Check sheet for the modelled part. Datum: model origin and axes. Units: mm. Face numbers are marked on the shaded views. A direction names the side the tool comes from. Round coordinates to 2 decimals unless told otherwise and drop trailing zeros. Write each loop counter-clockwise with the first axis right and the second up, starting at its lowest first coordinate (ties: lowest second). Pieces come first, ordered by that corner, then holes. Notation, with made-up numbers: M -22,18.25 L 24,18.25 A19 ccw 24,55.25 Z; hole C -37.75,54 d9. An arc over 180 degrees is marked long. Answer in a Markdown table with one row per item.
```python
from build123d import *

# Parameters (mm, degrees)
SKETCH_1_W          = 75
SKETCH_1_H          = 40
EXTRUDE_1_DEPTH     = 18
CHAMFER_1_SIZE      = 5
SKETCH_2_W          = 45
SKETCH_2_H          = 10
EXTRUDE_2_DEPTH     = 44.5
CHAMFER_2_SIZE      = 5
SKETCH_3_R          = 17.5
CUT_EXTRUDE_1_DEPTH = 101.778221854
SKETCH_4_R          = 1.5
CUT_EXTRUDE_2_DEPTH = 101.778221854
SKETCH_5_R          = 5
CUT_EXTRUDE_3_DEPTH = 6
SKETCH_6_R          = 2.75
CUT_EXTRUDE_4_DEPTH = 99.869863963


with BuildPart() as part:
    # 스케치1 → 보스-돌출1 (new body)
    with BuildSketch(Plane(origin=(0, 0, 0), x_dir=(1, 0, 0), z_dir=(0, 1, 0))):
        with Locations((37.5, 20)):
            Rectangle(SKETCH_1_W, SKETCH_1_H)
    extrude(amount=EXTRUDE_1_DEPTH)

    # 모따기1
    chamfer_1_edges = [part.edges().sort_by_distance(p)[0] for p in [
        (0, 9, -40),
        (75, 9, -40),
        (75, 9, 0),
        (0, 9, 0),
    ]]
    chamfer(chamfer_1_edges, length=CHAMFER_1_SIZE)

    # 스케치2 → 보스-돌출2 (add)
    with BuildSketch(Plane(origin=(0, 18, 0), x_dir=(1, 0, 0), z_dir=(0, 1, 0))):
        with Locations((37.5, 20)):
            Rectangle(SKETCH_2_W, SKETCH_2_H)
    extrude(amount=EXTRUDE_2_DEPTH)

    # 모따기2
    chamfer_2_edges = [part.edges().sort_by_distance(p)[0] for p in [
        (15, 62.5, -20),
        (60, 62.5, -20),
    ]]
    chamfer(chamfer_2_edges, length=CHAMFER_2_SIZE)

    # 스케치3 → 컷-돌출1 (cut, through all)
    with BuildSketch(Plane.XY.offset(-15)):
        with Locations((37.5, 40)):
            Circle(SKETCH_3_R)
    extrude(amount=-CUT_EXTRUDE_1_DEPTH, mode=Mode.SUBTRACT)

    # 스케치4 → 컷-돌출2 (cut, through all)
    with BuildSketch(Plane.XY.offset(-15)):
        with Locations((22.65, 54.85)):
            Circle(SKETCH_4_R)
        with Locations((52.35, 54.85)):
            Circle(SKETCH_4_R)
        with Locations((52.35, 25.15)):
            Circle(SKETCH_4_R)
        with Locations((22.65, 25.15)):
            Circle(SKETCH_4_R)
    extrude(amount=-CUT_EXTRUDE_2_DEPTH, mode=Mode.SUBTRACT)

    # 스케치5 → 컷-돌출3 (cut)
    with BuildSketch(Plane(origin=(0, 18, 0), x_dir=(1, 0, 0), z_dir=(0, 1, 0))):
        with Locations(Location((10, 32.5, 0), (0, 0, 270))):
            Circle(SKETCH_5_R)
        with Locations(Location((10, 7.5, 0), (0, 0, 270))):
            Circle(SKETCH_5_R)
        with Locations(Location((65, 7.5, 0), (0, 0, 270))):
            Circle(SKETCH_5_R)
        with Locations(Location((65, 32.5, 0), (0, 0, 270))):
            Circle(SKETCH_5_R)
    extrude(amount=-CUT_EXTRUDE_3_DEPTH, mode=Mode.SUBTRACT)

    # 스케치6 → 컷-돌출4 (cut, through all)
    with BuildSketch(Plane(origin=(0, 12, 0), x_dir=(1, 0, 0), z_dir=(0, 1, 0))):
        with Locations(Location((10, 7.5, 0), (0, 0, 270))):
            Circle(SKETCH_6_R)
        with Locations(Location((10, 32.5, 0), (0, 0, 270))):
            Circle(SKETCH_6_R)
        with Locations(Location((65, 7.5, 0), (0, 0, 270))):
            Circle(SKETCH_6_R)
        with Locations(Location((65, 32.5, 0), (0, 0, 270))):
            Circle(SKETCH_6_R)
    extrude(amount=-CUT_EXTRUDE_4_DEPTH, mode=Mode.SUBTRACT)


solid = part.part
```
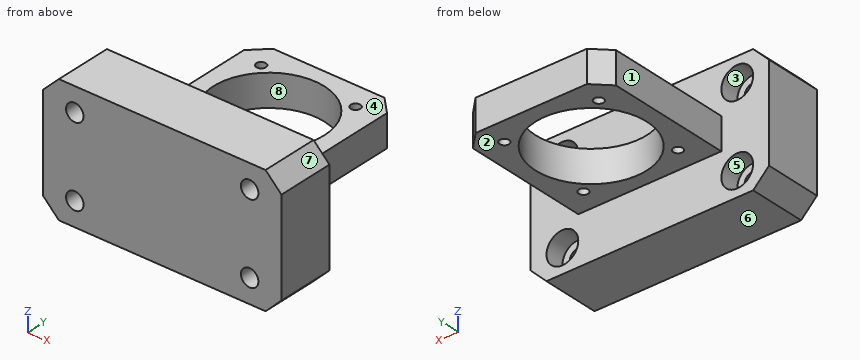
1. Access from +Z, -Z, +X, -X, +Y, -Y to the whole of each face (thin tool, end or side, straight path). Record for the marked faces 1, 2, 3 and 4.
Found:
| item | result |
|---|---|
| face 1 | +Z, -Z, -X, +Y |
| face 2 | -Z, +X, -X, +Y |
| face 3 | +Y |
| face 4 | +Z, +X, -X, +Y |
2. Section check C-C, the plane x = 10. Record the cut outline in (y, z).
Found:
| item | result |
|---|---|
| outline | M 0,-40 L 18,-40 L 18,-37.5 L 12,-37.5 L 12,-35.25 L 0,-35.25 Z; M 0,-29.75 L 12,-29.75 L 12,-27.5 L 18,-27.5 L 18,-12.5 L 12,-12.5 L 12,-10.25 L 0,-10.25 Z; M 0,-4.75 L 12,-4.75 L 12,-2.5 L 18,-2.5 L 18,0 L 0,0 Z |
3. Section check A-A, the plane y = 40. Record the cut outline in (x, z), and give its area (3 significant figures).
Found:
| item | result |
|---|---|
| outline | M 15,-25 L 20,-25 L 20,-15 L 15,-15 Z; M 55,-25 L 60,-25 L 60,-15 L 55,-15 Z |
| area | 100 mm2 |
4. Go/stop test with flat-tipped pins: pin 1 (5 mm diameter, centred on x = 22.65, y = 54.85, fed in from -Z); pin 2 (3 mm diameter, centred on y = 43, z = -20.5, fed in from -X); pin 3 (11 mm diameter, centred on x = 8.5, z = -32, fed in from +Y); pin 4 (1.8 mm diameter, centred on x = 22.65, y = 25.15, fed in from -Z). Record where each tip stops, or that it passes through.
Found:
| item | result |
|---|---|
| pin 1 | stops at z = -25 |
| pin 2 | stops at x = 15 |
| pin 3 | stops at y = 18 |
| pin 4 | passes through |
5. Section check D-D, the plane y = 14. Record the cut outline in (x, z).
Found:
| item | result |
|---|---|
| outline | M 0,-35 L 5,-40 L 70,-40 L 75,-35 L 75,-5 L 70,0 L 5,0 L 0,-5 Z; hole C 10,-32.5 d10; hole C 10,-7.5 d10; hole C 65,-32.5 d10; hole C 65,-7.5 d10 |
6. Scan lines: L1, parallel to X at y = 13.6, z = -7.5; L2, parallel to Z at x = 62.5, y = 12.5; L3, parallel to X at y = 9, z = -32. Record each from-to range of solid material in increasing order.
Found:
| item | result |
|---|---|
| L1 | x = 0 to 5, 15 to 60, 70 to 75 |
| L2 | z = -40 to -36.83, -28.17 to -11.83, -3.17 to 0 |
| L3 | x = 0 to 7.3, 12.7 to 62.3, 67.7 to 75 |
7. Section check B-B, the plane x = 37.5. Record the cut outline in (y, z), and give its area (3 significant figures).
Found:
| item | result |
|---|---|
| outline | M 0,-40 L 18,-40 L 18,-25 L 22.5,-25 L 22.5,-15 L 18,-15 L 18,0 L 0,0 Z; M 57.5,-25 L 62.5,-25 L 62.5,-15 L 57.5,-15 Z |
| area | 815 mm2 |
8. Draft check along X on the marked faces 5, 6, 7 and 8. Enter one of: +X half, -X half, draft (parallel to the pull), parting line (faces both ways), or undercut.
Found:
| item | result |
|---|---|
| face 5 | undercut |
| face 6 | draft |
| face 7 | +X half |
| face 8 | undercut |
